from build123d import *

# Parameters (mm, degrees)
CUT_EXTRUDE1_DEPTH = 20.32


with BuildPart() as part:
    # Sketch2 → Loft1 section 0
    with BuildSketch(Plane.XY.offset(50.8)):
        with BuildLine():
            Line((-14.298079416, 0), (-7.149039708, -12.3825))
            Line((-7.149039708, -12.3825), (7.149039708, -12.3825))
            Line((7.149039708, -12.3825), (14.298079416, 0))
            Line((14.298079416, 0), (7.149039708, 12.3825))
            Line((7.149039708, 12.3825), (-7.149039708, 12.3825))
            Line((-7.149039708, 12.3825), (-14.298079416, 0))
        make_face()
    # Sketch1 → Loft1 section 1
    with BuildSketch(Plane.XY):
        with BuildLine():
            Line((11.438463533, 0), (5.719231767, 9.906))
            Line((5.719231767, 9.906), (-5.719231767, 9.906))
            Line((-5.719231767, 9.906), (-11.438463533, 0))
            Line((-11.438463533, 0), (-5.719231767, -9.906))
            Line((-5.719231767, -9.906), (5.719231767, -9.906))
            Line((5.719231767, -9.906), (11.438463533, 0))
        make_face()
    loft()

    # Sketch4 → Cut-Extrude1 (cut)
    with BuildSketch(Plane(origin=(0, 0, 0), x_dir=(-1, 0, 0), z_dir=(0, 0, -1))):
        Polygon((-9.45872946, 3.429), (9.45872946, 3.429), (15.693203295, 3.429), (15.693203295, -3.175), (9.605376429, -3.175), (-9.605376429, -3.175), (-15.693203295, -3.175), (-15.693203295, 3.429), align=None)
    extrude(amount=-CUT_EXTRUDE1_DEPTH, mode=Mode.SUBTRACT)


solid = part.part
The listing builds one solid part. Answer for the finished solid, in the listing's coordinates (mm). A direction names the side the tool comes from. Round coordinates to 2 decimals unless told otherwise and drop trailing zeros. Answer in a Markdown table with one row per item. Add a question column.
1) Determine the mould class of faces 3 (the face through (0, 0, 20.32)), 4 (the face through (0, -3.175, 10)), 5 (the face through (0, 7, 0)) for opening direction Y: pulls with the +Y half, pulls with the -Y half, needs draft (parallel to the pull), parting line crosses it, or undercut.
2) Which of the six approach directions +Z, -Z, +X, -X, +Y, -Y give full straight-line access (tool end or side, diameter ignored) to faces 1 (the face through (0, -7, 0)), 2 (the face through (0, 3.429, 10))?
3) Consider line 1 along Y through (x, z) = (6.75, 13) (3 decimals); line 2 along Y through (x, z) = (-5, 8) (3 decimals); line 3 along Z through (x, y) = (-0.25, 0). Determine where each line is inside the solid, lowest interval first. Write a range as from..to.
4) Flat-ended cylindrical pins translate along their axes: pin 1 Ø1.5 at (x, y) = (-5, -8.5) entering from -Z; pin 2 Ø3 at (y, z) = (-8, 8.5) entering from -X; pin 3 Ø4 at (y, z) = (4.5, 31.5) entering from +X; pin 4 Ø16.5 at (x, z) = (2, 13) entering from -Y. Find the tip coordinate at first contact, or state that the pin passes through.
Findings below:
| question | item | result |
|---|---|---|
| 1 | face 3 | undercut |
| 1 | face 4 | undercut |
| 1 | face 5 | needs draft |
| 2 | face 1 | -Z, +X, -X, +Y, -Y |
| 2 | face 2 | -Z, +X, -X |
| 3 | line 1 | y = -9.388..-3.175, 3.429..9.388 |
| 3 | line 2 | y = -10.296..-3.175, 3.429..10.296 |
| 3 | line 3 | z = 20.32..50.8 |
| 4 | pin 1 | stops at z = 0 |
| 4 | pin 2 | stops at x = -8.17 |
| 4 | pin 3 | stops at x = 11.77 |
| 4 | pin 4 | stops at y = -10.94 |
